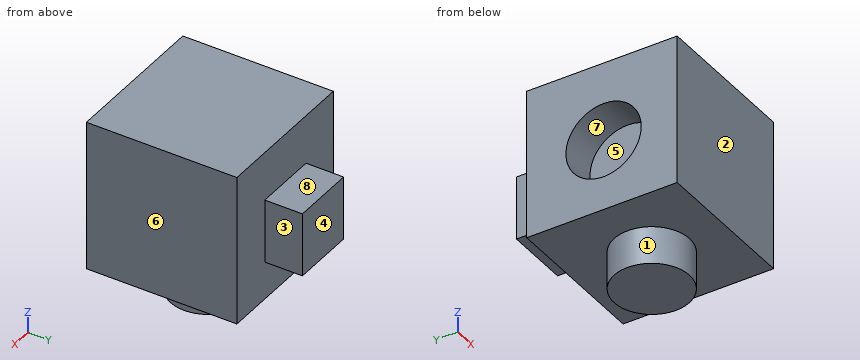
from build123d import *

# Parameters (mm, degrees)
F0_W     = 50.8
F0_H     = 50.8
F1_DEPTH = 50.8
F2_W     = 21.704316
F2_H     = 21.507005
F3_DEPTH = 12.7
F4_R     = 12.7
F5_DEPTH = 12.7
F6_R     = 12.7
F7_DEPTH = 12.7


with BuildPart() as f1:
    # F0 (on Front) → F1 (new body)
    with BuildSketch(Plane.XZ):
        with Locations((-25.4, 25.4)):
            Rectangle(F0_W, F0_H)
    extrude(amount=F1_DEPTH)

    # F2 (on Front) → F3 (join)
    with BuildSketch(Plane.XZ):
        with Locations((-25.5519, 23.57878)):
            Rectangle(F2_W, F2_H)
    extrude(amount=-F3_DEPTH)

    # F4 (on face) → F5 (cut)
    with BuildSketch(Plane(origin=(-50.8, 0, 0), x_dir=(0, -1, 0), z_dir=(-1, 0, 0))):
        with Locations((25.946522, 24.07206)):
            Circle(F4_R)
    extrude(amount=-F5_DEPTH, mode=Mode.SUBTRACT)

    # F6 (on face) → F7 (join)
    with BuildSketch(Plane(origin=(0, 0, 0), x_dir=(1, 0, 0), z_dir=(0, 0, -1))):
        with Locations((-25.551898, 26.044877)):
            Circle(F6_R)
    extrude(amount=F7_DEPTH)


solid = f1.part
Here's how the part is built. I have some questions about the finished solid (model axes, mm). Face numbers are marked on the shaded views. A direction names the side the tool comes from. Coordinates: 2 decimals unless noted, no trailing zeros. Write each loop counter-clockwise with the first axis right and the second up, starting at its lowest first coordinate (ties: lowest second). Pieces come first, ordered by that corner, then holes.
Item 1: If we mould it in two halves opening along Z, with no side actions, what happens to the marked faces 6, 7 and 8? For each: +Z half, -Z half, draft (parallel to the pull), parting line (faces both ways), or undercut.
Item 2: I want a section at C-C on y = -7.5. Write out the boundary of the cut face in (x, z).
Item 3: I want a section at B-B on x = -16.5. Write out the boundary of the cut face in (y, z).
Item 4: If I drill on line 1 (Y direction, x = -7, z = 6); line 2 (Z direction, x = -40, y = -42.5); line 3 (Y direction, x = -45.5, z = 13), over which ranges is the centre line in solid material (lowest first)?
Item 5: On a 3-axis mill with a long thin cutter (end or side, diameter ignored), from which of +Z, -Z, +X, -X, +Y, -Y can I reach the whole of each face in a straight line? I mean the marked faces 1, 2, 3, 4 and 5. Say none if no direction works.
Item 6: I want a section at D-D on x = -44.5. Write out the boundary of the cut face in (y, z).
Item 7: Will these pins go through, and if not, where does the flat tip stop? pin 1 (5 mm diameter, centred on x = -38, z = 34.5, fed in from +Y); pin 2 (4 mm diameter, centred on x = -26, y = 5, fed in from -Z); pin 3 (6.5 mm diameter, centred on y = 6, z = 22, fed in from +X); pin 4 (1 mm diameter, centred on y = -30.5, z = 13, fed in from -X).
Item 8: I want a section at A-A on z = 31. Write out the boundary of the cut face in (x, y), and give its area (3 significant figures).
Findings below:
1. face 6: draft
1. face 7: undercut
1. face 8: +Z half
2. outline: (-50.8, 0) - (0, 0) - (0, 50.8) - (-50.8, 50.8) - close
3. outline: (-50.8, 0) - (-34.95, 0) - (-34.95, -12.7) - (-17.14, -12.7) - (-17.14, 0) - (0, 0) - (0, 12.83) - (12.7, 12.83) - (12.7, 34.33) - (0, 34.33) - (0, 50.8) - (-50.8, 50.8) - close
4. line 1: y = -50.8 to 0
4. line 2: z = 0 to 50.8
4. line 3: y = -50.8 to -32.17, -19.73 to 0
5. face 1: -Z
5. face 2: +Z, -Z, +X, -X, -Y
5. face 3: +Z, -Z, +X, +Y
5. face 4: +Z, -Z, +X, -X, +Y
5. face 5: -X
6. outline: (-50.8, 0) - (0, 0) - (0, 50.8) - (-50.8, 50.8) - close; hole circle Ø25.4 at (-25.95, 24.07)
7. pin 1: stops at y = 12.7
7. pin 2: stops at z = 12.83
7. pin 3: stops at x = -14.7
7. pin 4: stops at x = -38.1
8. outline: (-50.8, -50.8) - (0, -50.8) - (0, 0) - (-14.7, 0) - (-14.7, 12.7) - (-36.4, 12.7) - (-36.4, 0) - (-50.8, 0) - (-50.8, -15.3) - (-38.1, -15.3) - (-38.1, -36.59) - (-50.8, -36.59) - close
8. area: 2,590 mm2
